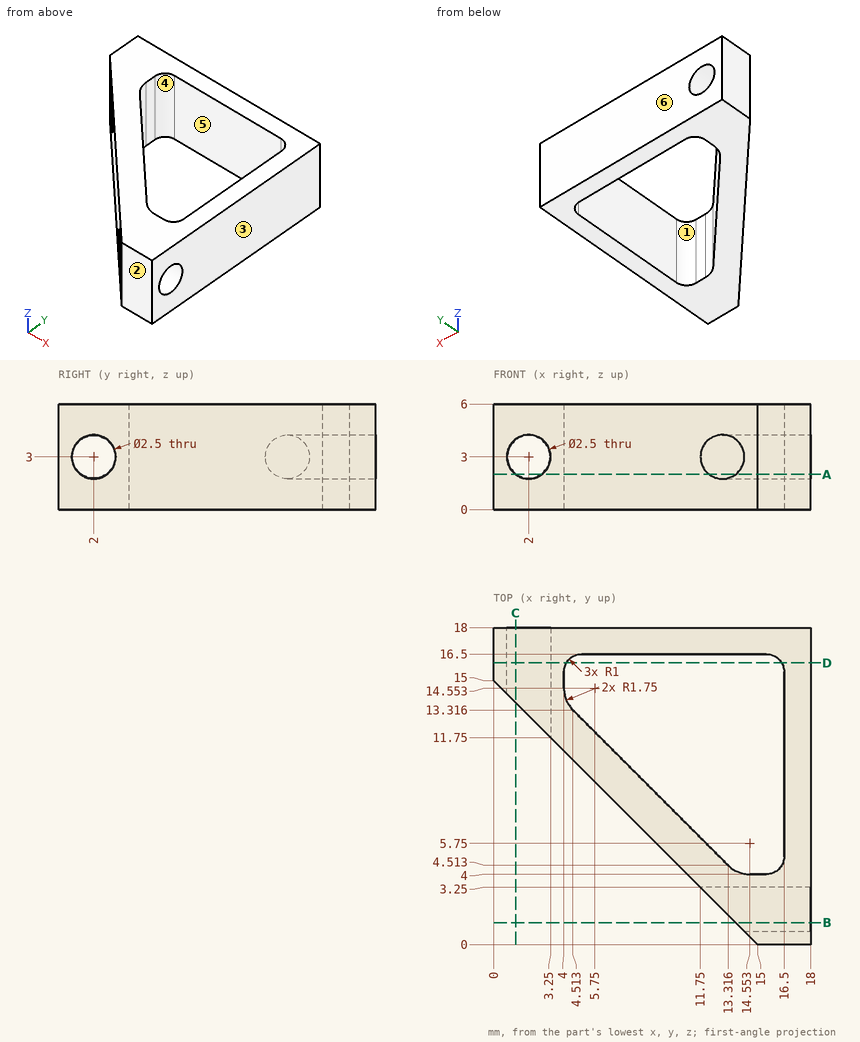
Geometry: see drawing. Coordinates: mm, zero at the bounding-box minimum. A direction names the side the tool comes from. Round coordinates to 2 decimals unless told otherwise and drop trailing zeros. Loops run counter-clockwise (first coordinate to the right, second up) from the corner with the lowest first, then second, coordinate; pieces in that order, holes last. Notation, with made-up numbers: (69.25, -35) - (99.25, -35) arc R18 ccw to (99.25, -9) - close; hole circle Ø4 at (87.25, -13.75). An arc over 180 degrees is marked (long way). Use CSV: the item, a comma, the result in double quotes.
Q1. Pin query (flat end, axial travel): pin 1 Ø3 at (y, z) = (2, 3) entering from -X; pin 2 Ø3 at (x, z) = (11.5, 5) entering from -Y; pin 3 Ø1.8 at (y, z) = (9, 3.5) entering from -X. Return the tip coordinate at first contact, or that it passes through.
Reported:
pin 1,"x = 11.5"
pin 2,"y = 2"
pin 3,"x = 5.1"
Q2. Section query A-A, the plane z = 2. Give the number of separate pieces and of enclosed holes in the cut face.
Reported:
separate pieces,"3"
enclosed holes,"1"
Q3. Section query B-B, the plane y = 1.25. Output: boundary loops of the cut face in (x, z), then the cut area to 3 significant figures.
Reported:
outline,"(13.75, 0) - (18, 0) - (18, 2) - (13.75, 2) - close; (13.75, 4) - (18, 4) - (18, 6) - (13.75, 6) - close"
area,"17.0 mm^2"
Q4. Reachability of the marked faces 5 and 6 from +Z, -Z, +X, -X, +Y, -Y: full face, straight path, thin tool, end or side. Return the list, or none.
Reported:
face 5,"+Z, -Z"
face 6,"+Z, -Z, +X, -X, +Y"
Q5. Ray query, line 1 along Z through (x, y) = (16.25, 2); line 2 along X through (y, z) = (14.5, 5.75); line 3 along Y through (x, z) = (12, 4). Return the intervals inside material, ascending.
Reported:
line 1,"0 to 1.75, 4.25 to 6"
line 2,"0.5 to 4, 16.5 to 18"
line 3,"3 to 5.83, 16.5 to 18"
Q6. Mould query, pull axis X, two halves, no side actions, for the marked faces 1, 2, 3 and 4. Classes: pulls with the +X half, pulls with the -X half, needs draft (parallel to the pull), parting line crosses it, or undercut.
Reported:
face 1,"undercut"
face 2,"needs draft"
face 3,"pulls with the +X half"
face 4,"undercut"
Q7. Section query D-D, the plane y = 16. Output: boundary loops of the cut face in (x, z).
Reported:
outline,"(0, 0) - (4.13, 0) - (4.13, 6) - (0, 6) - close; (16.37, 0) - (18, 0) - (18, 6) - (16.37, 6) - close; hole circle Ø2.5 at (2, 3)"
